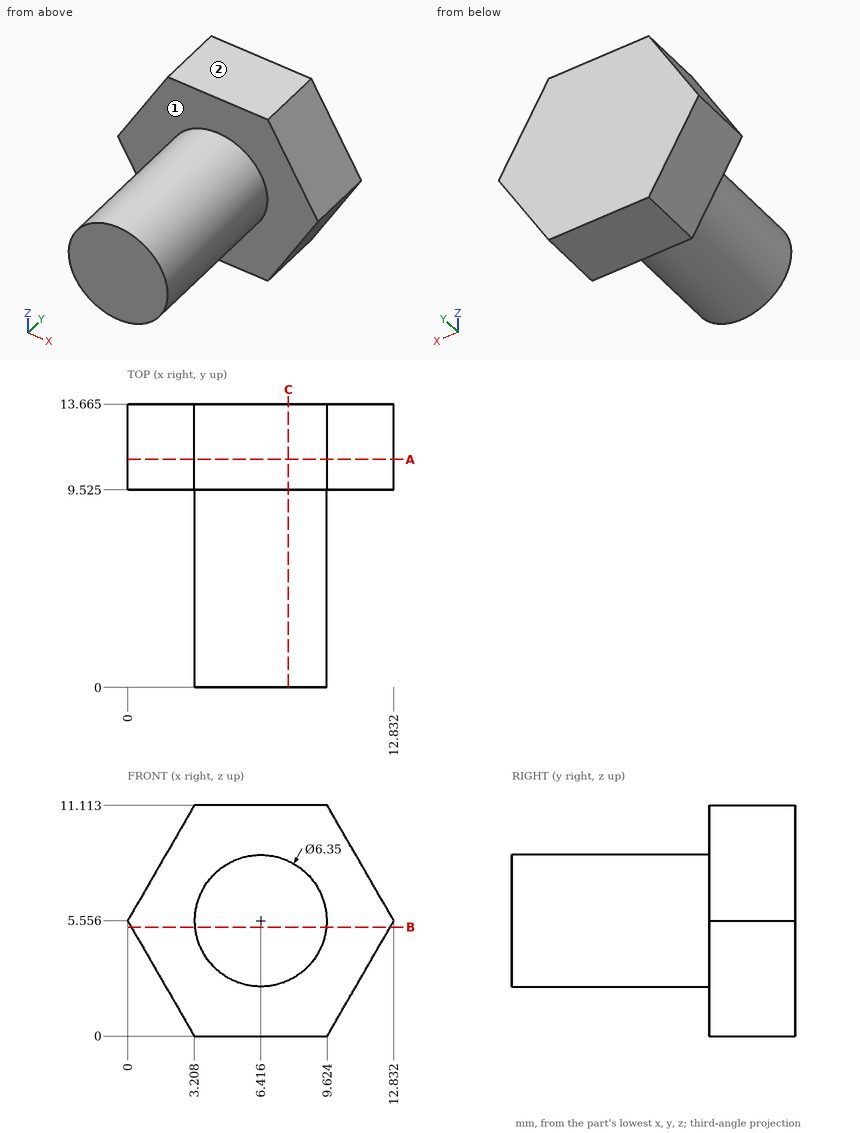
Study the drawing (mm; zero at the part's minimum x, y, z) and answer. A direction names the side the tool comes from. Give positions to 0.01 mm unless a question says otherwise; leave off trailing zeros. Write each loop counter-clockwise with the first axis right and the second up, starting at its lowest first coordinate (ties: lowest second). Pieces come first, ordered by that corner, then holes. Notation, with made-up numbers: M 4.25,10 L 63.25,10 A18 cw 63.25,16 Z; hole C -24.5,38 d5. An arc over 180 degrees is marked long. Put each result on its own line as item: value. Start each with the question number.
1. Each of these flat-tipped pins is pushed along its axis until it touches: pin 1 Ø3 at (y, z) = (6, 3) entering from -X; pin 2 Ø1 at (y, z) = (4.5, 9) entering from +X (1 decimal); pin 3 Ø5 at (y, z) = (5, 3.5) entering from -X; pin 4 Ø5.5 at (x, z) = (4.5, 6) entering from -Y. Where does it stop, or does it pass through?
2. The part is cut by section A-A, the plane y = 11. Give the vertices of the cut face in (x, z), and give its area (3 significant figures).
3. The part is cut by section B-B, the plane z = 5.25. Give the vertices of the cut face in (x, y) (1 decimal), and give its area (3 significant figures).
4. Consider line 1 along Y through (x, z) = (0.75, 6.5) (1 decimal); line 2 along X through (y, z) = (10.75, 10.5) (1 decimal); line 3 along Z through (x, y) = (6.5, 6). Determine where each line is inside the solid, lowest interval first.
5. The part is cut by section C-C, the plane x = 7.75. Give the vertices of the cut face in (y, z) (1 decimal).
6. Which of the six approach directions +Z, -Z, +X, -X, +Y, -Y give full straight-line access (tool end or side, diameter ignored) to the marked faces 1 and 2?
Final values:
1. pin 1: stops at x = 3.42
1. pin 2: stops at x = 7.6
1. pin 3: stops at x = 3.24
1. pin 4: stops at y = 0
2. outline: M 0,5.56 L 3.21,0 L 9.62,0 L 12.83,5.56 L 9.62,11.11 L 3.21,11.11 Z
2. area: 107 mm²
3. outline: M 0.2,9.5 L 3.3,9.5 L 3.3,0 L 9.6,0 L 9.6,9.5 L 12.7,9.5 L 12.7,13.7 L 0.2,13.7 Z
3. area: 112 mm²
4. line 1: y = 9.5 to 13.7
4. line 2: x = 2.9 to 10
4. line 3: z = 2.38 to 8.73
5. outline: M 0,2.7 L 9.5,2.7 L 9.5,0 L 13.7,0 L 13.7,11.1 L 9.5,11.1 L 9.5,8.4 L 0,8.4 Z
6. face 1: -Y
6. face 2: +Z, +X, -X, +Y, -Y
